Can you work these out from the model? Positions are in its coordinate system, mm. A direction names the side the tool comes from. Give positions to 0.01 mm unless a question says otherwise; leave off trailing zeros. Write each loop counter-clockwise with the first axis right and the second up, starting at its lowest first coordinate (ties: lowest second). Pieces come first, ordered by that corner, then holes. Notation, with made-up numbers: (-5, 5) - (45, 5) arc R12 ccw to (45, 13) - close; hole circle Ø4 at (-10.5, 66.25). An arc over 180 degrees is marked (long way). Use a Markdown table: item, result. Add a question column.
```python
from build123d import *

# Parameters (mm, degrees)
SKETCH1_W                = 13
SKETCH1_H                = 8
BOSS_EXTRUDE1_DEPTH      = 7
BOSS_EXTRUDE2_DEPTH      = 2
BOSS_EXTRUDE2_DEPTH_BACK = 50
SKETCH2_W                = 10
SKETCH2_H                = 17
BOSS_EXTRUDE3_REACH      = 56.9
SKETCH3_W                = 17
SKETCH3_H                = 2
FILLET4_R                = 5
FILLET3_R                = 2
SKETCH4_W                = 17
SKETCH4_H                = 7
CUT_EXTRUDE1_DEPTH       = 7
BOSS_EXTRUDE4_DEPTH      = 13
SHELL1_START             = -13
SHELL1_OUTLINE_W         = 6
SHELL1_OUTLINE_H         = 48
SHELL1_DEPTH             = 13
SHELL1_START_2           = -11
SHELL1_2_DEPTH           = 9
CUT_EXTRUDE2_REACH       = 55.151
SKETCH6_R                = 4.9
CHAMFER1_SIZE            = 0.5
CUT_EXTRUDE3_REACH       = 56.9
SKETCH7_R                = 2.75
SKETCH8_R                = 1.75
CUT_EXTRUDE4_DEPTH       = 55.899908953
CUT_EXTRUDE5_REACH       = 56.9
CUT_EXTRUDE6_START       = -12.6
CUT_EXTRUDE6_DEPTH       = 12.6
CHAMFER2_SIZE            = 0.5


# Read off the part's stored shape, not the designer's step: Shell1
# Some blends are built 0.0001 mm under size
with BuildPart() as part:
    # Sketch1 → Boss-Extrude1 (new body)
    with BuildSketch(Plane(origin=(0, 0, 0), x_dir=(0, 0, -1), z_dir=(1, 0, 0))):
        with Locations((6.5, 4)):
            Rectangle(SKETCH1_W, SKETCH1_H)
    extrude(amount=BOSS_EXTRUDE1_DEPTH)

    # Sketch2 → Boss-Extrude2 (add, two sides: drawn at the far end of the back side and taken through both)
    with BuildSketch(Plane(origin=(0, 0, 0), x_dir=(-1, 0, 0), z_dir=(0, -1, 0)).offset(-BOSS_EXTRUDE2_DEPTH_BACK)):
        with Locations((5, 6.5)):
            Rectangle(SKETCH2_W, SKETCH2_H)
    extrude(amount=BOSS_EXTRUDE2_DEPTH + BOSS_EXTRUDE2_DEPTH_BACK)

    # Sketch3 → Boss-Extrude3 (add, up to next)
    with BuildSketch(Plane(origin=(7, 0, 0), x_dir=(0, 0, -1), z_dir=(1, 0, 0)), mode=Mode.PRIVATE) as boss_extrude3_sk1:
        with Locations((6.5, 9)):
            Rectangle(SKETCH3_W, SKETCH3_H)
    boss_extrude3_tool1 = extrude(boss_extrude3_sk1.sketch, amount=-BOSS_EXTRUDE3_REACH, mode=Mode.PRIVATE) - part.part
    add(boss_extrude3_tool1.solids().sort_by_distance((7, 9, -6.5))[0])

    # Fillet4
    fillet4_edges = [part.edges().sort_by_distance(p)[0] for p in [
        (0, 10, -6.5),
    ]]
    fillet(fillet4_edges, radius=FILLET4_R)

    # Fillet3
    fillet3_edges = [part.edges().sort_by_distance(p)[0] for p in [
        (-5, 50, -15),
        (-10, 50, -6.5),
        (-5, 50, 2),
        (0, 50, -6.5),
        (-10, 24, 2),
        (-5, -2, 2),
        (-10, 24, -15),
        (-10, -2, -6.5),
        (-5, -2, -15),
        (6, 10, -15),
        (1.464466094, 11.464466094, -15),
        (6, 10, 2),
        (1.464466094, 11.464466094, 2),
        (0, 32.5, -15),
        (0, 32.5, 2),
    ]]
    fillet(fillet3_edges, radius=FILLET3_R - 0.0001)  # a hair under: the kernel refuses the full size

    # Sketch4 → Cut-Extrude1 (cut)
    with BuildSketch(Plane(origin=(7, 0, 0), x_dir=(0, 0, -1), z_dir=(1, 0, 0))):
        with Locations((6.5, 11.5)):
            Rectangle(SKETCH4_W, SKETCH4_H)
    extrude(amount=-CUT_EXTRUDE1_DEPTH, mode=Mode.SUBTRACT)

    # Sketch5 → Boss-Extrude4 (add)
    with BuildSketch(Plane(origin=(0, 0, -13), x_dir=(-1, 0, 0), z_dir=(0, 0, -1))):
        with BuildLine():
            Line((0, 8), (-5, 8))
            ThreePointArc((-5, 8), (-2.288252998, 8.546595612), (0, 10.101020514))
            Line((0, 10.101020514), (0, 8))
        make_face()
    extrude(amount=-BOSS_EXTRUDE4_DEPTH)

    # Shell1 outline → Shell1 (cut)
    with BuildSketch(Plane.XY.offset(SHELL1_START)):
        with Locations((-5, 24)):
            Rectangle(SHELL1_OUTLINE_W, SHELL1_OUTLINE_H)
    extrude(amount=SHELL1_DEPTH, mode=Mode.SUBTRACT)

    # Shell1 2 outline → Shell1 2 (cut)
    with BuildSketch(Plane.XY.offset(SHELL1_START_2)):
        with BuildLine():
            Line((-2, 2), (7, 2))
            Line((7, 2), (7, 6))
            Line((7, 6), (5, 6))
            ThreePointArc((5, 6), (1.121320343, 6.878679656), (-2, 9.343145751))
            Line((-2, 9.343145751), (-2, 2))
        make_face()
    extrude(amount=SHELL1_2_DEPTH, mode=Mode.SUBTRACT)

    # Sketch6 → Cut-Extrude2 (cut, up to next)
    with BuildSketch(Plane(origin=(0, 0, 0), x_dir=(0, 0, -1), z_dir=(1, 0, 0)), mode=Mode.PRIVATE) as cut_extrude2_sk1:
        with Locations((6.5, 36.75)):
            Circle(SKETCH6_R)
    cut_extrude2_tool1 = extrude(cut_extrude2_sk1.sketch, amount=-CUT_EXTRUDE2_REACH, mode=Mode.PRIVATE) & part.part
    add(cut_extrude2_tool1.solids().sort_by_distance((0, 36.75, -6.5))[0], mode=Mode.SUBTRACT)

    # Chamfer1
    chamfer1_edges = [part.edges().sort_by_distance(p)[0] for p in [
        (0, 36.75, -1.6),
    ]]
    chamfer(chamfer1_edges, length=CHAMFER1_SIZE)

    # Cut-Extrude3: up to this face of the body (flat: up to its plane)
    cut_extrude3_end = Plane(part.part.faces().sort_by_distance((-8, 24, -6.5))[0])
    # Sketch7 → Cut-Extrude3 (cut, up to the picked face)
    with BuildSketch(Plane(origin=(7, 0, 0), x_dir=(0, 0, -1), z_dir=(1, 0, 0)), mode=Mode.PRIVATE) as cut_extrude3_sk1:
        with Locations((9.5, 4)):
            Circle(SKETCH7_R)
    cut_extrude3_tool1 = split(extrude(cut_extrude3_sk1.sketch, amount=-CUT_EXTRUDE3_REACH, mode=Mode.PRIVATE), bisect_by=cut_extrude3_end, keep=Keep.BOTH, mode=Mode.PRIVATE)
    add(cut_extrude3_tool1.solids().sort_by(Axis((7, 4, -9.5), (-1, 0, 0)))[0], mode=Mode.SUBTRACT)

    # Sketch8 → Cut-Extrude4 (cut, through all)
    with BuildSketch(Plane(origin=(7, 0, 0), x_dir=(0, 0, -1), z_dir=(1, 0, 0))):
        with Locations((9.5, 4)):
            Circle(SKETCH8_R)
    extrude(amount=-CUT_EXTRUDE4_DEPTH, mode=Mode.SUBTRACT)

    # Cut-Extrude5: up to this face of the body (flat: up to its plane)
    cut_extrude5_end = Plane(part.part.faces().sort_by_distance((0, 23.174375266, -6.49999999))[0])
    # Sketch9 → Cut-Extrude5 (cut, up to the picked face)
    with BuildSketch(Plane(origin=(7, 0, 0), x_dir=(0, 0, -1), z_dir=(1, 0, 0)), mode=Mode.PRIVATE) as cut_extrude5_sk1:
        Polygon((0, 10.101020514), (0.2, 10.101020514), (0.2, 0.2), (12.8, 0.2), (12.8, 10.101020514), (13, 10.101020514), (13, 0), (0, 0), align=None)
    cut_extrude5_tool1 = split(extrude(cut_extrude5_sk1.sketch, amount=-CUT_EXTRUDE5_REACH, mode=Mode.PRIVATE), bisect_by=cut_extrude5_end, keep=Keep.BOTH, mode=Mode.PRIVATE)
    add(cut_extrude5_tool1.solids().sort_by(Axis((7, 9.93639, -0.1), (-1, 0, 0)))[0], mode=Mode.SUBTRACT)

    # Sketch10 → Cut-Extrude6 (cut)
    with BuildSketch(Plane.XY.offset(-0.2).offset(CUT_EXTRUDE6_START)):
        with BuildLine():
            Line((7, 8), (5, 8))
            ThreePointArc((5, 8), (2.288252998, 8.546595612), (0, 10.101020514))
            Line((0, 10.101020514), (0, 9.819266461))
            ThreePointArc((0, 9.819266461), (2.303825069, 8.32387532), (5, 7.8))
            Line((5, 7.8), (7, 7.8))
            Line((7, 7.8), (7, 8))
        make_face()
    extrude(amount=CUT_EXTRUDE6_DEPTH, mode=Mode.SUBTRACT)

    # Chamfer2
    # the kernel refuses this chamfer: 0.5 mm, written as the material it takes off along each edge
    with BuildSketch(Plane(origin=(7, 4, -9.5), x_dir=(0, 0.33829869190957257, 0.9410387850945741), z_dir=(0, -0.9410387850945741, 0.33829869190957257))) as chamfer2_piece_1:
        Polygon((2.75 + CHAMFER2_SIZE, 0), (2.75, CHAMFER2_SIZE), (2.75, 0), align=None)
    revolve(axis=Axis((7, 4, -9.5), (-1, 0, 0)), revolution_arc=320.453489915, mode=Mode.SUBTRACT)
    with BuildSketch(Plane(origin=(7, 0.2, 1.085841494), x_dir=(-0.9996219169112968, -0.027495876610586403, 0), z_dir=(0, 0, -1))) as chamfer2_piece_2:
        Polygon((CHAMFER2_SIZE * 0.999621916911, CHAMFER2_SIZE * 0.0274958766106), (-CHAMFER2_SIZE * 0.0274958766106, CHAMFER2_SIZE * 0.999621916911), (0, 0), align=None)
    extrude(amount=15.171682988, mode=Mode.SUBTRACT)
    with BuildSketch(Plane(origin=(7, 9.085841494, -0.2), x_dir=(-0.9996219169112968, 0, 0.027495876610586403), z_dir=(0, -1, 0)), Plane(origin=(7, -1.085841494, -12.8), x_dir=(-0.9996219169112968, 0, -0.027495876610585647), z_dir=(0, 1, 0))) as chamfer2_piece_3:
        Polygon((CHAMFER2_SIZE * 0.999621916911, CHAMFER2_SIZE * 0.0274958766106), (-CHAMFER2_SIZE * 0.0274958766106, CHAMFER2_SIZE * 0.999621916911), (0, 0), align=None)
    extrude(amount=10.171682988, mode=Mode.SUBTRACT)
    with BuildSketch(Plane(origin=(7, 7.8, -14.085841494), x_dir=(0.027495876610585647, -0.9996219169112968, 0), z_dir=(0, 0, 1))) as chamfer2_piece_4:
        Polygon((CHAMFER2_SIZE * 0.999621916911, -CHAMFER2_SIZE * 0.0274958766106), (-CHAMFER2_SIZE * 0.0274958766106, -CHAMFER2_SIZE * 0.999621916911), (0, 0), align=None)
    extrude(amount=15.171682988, mode=Mode.SUBTRACT)


solid = part.part
```
Q1. If we mould it in two halves opening along X, with no side actions, what happens to faces 6 (the flat face through (-10, 24, -6)), 7 (the conical face through (6.635, 4.1, -12.384)), 8 (the flat face through (-8, 24, -7))? For each: released by +X, released by -X, zero draft, split by the parting line, or undercut.
Q2. If I drill on probe 1 along X at (y, z) = (47, -6.75); probe 2 along Y at (x, z) = (-7, -12.5); probe 3 along Z at (x, y) = (-3.5, 25), over which ranges is the centre line in solid material (lowest first)? Write a range as [from, to].
Q3. Suppose I cut it at A-A (x = -4.5). Please give me the cut outline in (y, z).
Q4. Suppose I cut it at C-C (y = 36.75). Please give me the cut outline in (x, z), and give its area (3 significant figures).
Q5. Suppose I cut it at D-D (z = -9.5). Give the number of separate pieces and of enclosed holes in the cut face, and give its area (3 significant figures).
Q6. I'm going to push flat-ended pins straight in: P1, Ø3.5, axis at x = 4.5, z = -5.5, coming from the -Y side; P2, Ø2, axis at x = 3.5, y = 6, coming from the +Z side; P3, Ø7, axis at y = 4, z = -9.5, coming from the +X side; P4, Ø1.7, axis at x = 1, z = -4.5, coming from the +Y side. Where does each tip first touch, or does it pass through?
Q7. Suppose I cut it at B-B (y = 4). Please give me the cut outline in (x, z) (3 decimals), and give its area (3 significant figures).
Q8. On a 3-axis mill with a long thin cutter (end or side, diameter ignored), from which of +Z, -Z, +X, -X, +Y, -Y can I reach the whole of each face in a straight line? I mean faces 1 (the flat face through (3, 4, -0.2)), 2 (the flat face through (6, 6, -5)), 3 (the flat face through (-5, 24, -13)), 4 (the flat face through (3, 4, -12.8)), 5 (the flat face through (6, 7.8, -7)). Say none if no direction works.
Derived:
| question | item | result |
|---|---|---|
| 1 | face 6 | released by -X |
| 1 | face 7 | released by +X |
| 1 | face 8 | undercut |
| 2 | probe 1 | [-10, -8], [-2, 0] |
| 2 | probe 2 | [-2, 0], [48, 50] |
| 2 | probe 3 | [-15, -13], [0, 2] |
| 3 | outline | (-2, -13) arc R2 ccw to (0, -15) - (48, -15) arc R2 ccw to (50, -13) - (50, 0) arc R2 ccw to (48, 2) - (0, 2) arc R2 ccw to (-2, 0) - close; hole (0, -13) - (48, -13) - (48, 0) - (0, 0) - close |
| 4 | outline | (-10, -13) arc R2 ccw to (-8, -15) - (-2, -15) arc R2 ccw to (0, -13) - (0, -11.9) - (-0.5, -11.4) - (-2, -11.4) - (-2, -13) - (-8, -13) - (-8, 0) - (-2, 0) - (-2, -1.6) - (-0.5, -1.6) - (0, -1.1) - (0, 0) arc R2 ccw to (-2, 2) - (-8, 2) arc R2 ccw to (-10, 0) - close |
| 4 | area | 68.7 mm² |
| 5 | separate pieces | 3 |
| 5 | enclosed holes | 0 |
| 5 | area | 209 mm² |
| 6 | P1 | y = 0.2 |
| 6 | P2 | z = -0.2 |
| 6 | P3 | x = 7 |
| 6 | P4 | y = 9.68 |
| 7 | outline | (-10, -13) arc R2 ccw to (-8, -15) - (0, -15) - (0, -12.8) - (6.5, -12.8) - (6.775, -12.525) - (6.5, -12.25) - (-2, -12.25) - (-2, -13) - (-8, -13) - (-8, -11.25) - (-10, -11.25) - close; (-10, -7.75) - (-8, -7.75) - (-8, 0) - (-2, 0) - (-2, -2) - (7, -2) - (7, -0.7) - (6.5, -0.2) - (0, -0.2) - (0, 2) - (-8, 2) arc R2 ccw to (-10, 0) - close |
| 7 | area | 78.9 mm² |
| 8 | face 1 | +Z, +X, +Y, -Y |
| 8 | face 2 | +X |
| 8 | face 3 | none |
| 8 | face 4 | -Z, +X, +Y, -Y |
| 8 | face 5 | +Z, -Z, +X, +Y |
